```python
from build123d import *

# Parameters (mm, degrees)
CYLINDER_R        = 3.15
CYLINDER_DEPTH    = 10
CYLINDER001_R     = 6.5
CYLINDER001_DEPTH = 3
BOX_W             = 24
BOX_H             = 8
BOX_DEPTH         = 20
CHAMFER_SIZE      = 5
BOX001_W          = 7.8
BOX001_H          = 1
BOX001_DEPTH      = 20
FILLET_R          = 1
CHAMFER001_SIZE   = 0.4


with BuildPart() as cylinder:
    # Cylinder → Cylinder (new body)
    with BuildSketch(Plane(origin=(0, 0, 10), x_dir=(1, 0, 0), z_dir=(0, 1, 0))):
        Circle(CYLINDER_R)
    extrude(amount=CYLINDER_DEPTH)


with BuildPart() as fusion:
    # Cylinder001 → Cylinder001 (new body)
    with BuildSketch(Plane(origin=(0, 0, 10), x_dir=(1, 0, 0), z_dir=(0, 1, 0))):
        Circle(CYLINDER001_R)
    extrude(amount=CYLINDER001_DEPTH)

    # Fusion: union Cylinder
    add(cylinder.part)


with BuildPart() as chamfer_body:
    # Box → Box (new body)
    with BuildSketch(Plane(origin=(-12, 0, 0), x_dir=(1, 0, 0), z_dir=(0, 0, 1))):
        with Locations((12, 4)):
            Rectangle(BOX_W, BOX_H)
    extrude(amount=BOX_DEPTH)

    # Chamfer
    chamfer_edges = [chamfer_body.edges().sort_by_distance(p)[0] for p in [
        (-12, 4, 20),
        (12, 4, 20),
    ]]
    chamfer(chamfer_edges, length=CHAMFER_SIZE)


with BuildPart() as chamfer001:
    # Box001 → Box001 (new body)
    with BuildSketch(Plane(origin=(-3.9, 8, 0), x_dir=(1, 0, 0), z_dir=(0, 0, 1))):
        with Locations((3.9, 0.5)):
            Rectangle(BOX001_W, BOX001_H)
    extrude(amount=BOX001_DEPTH)

    # Fusion001: union Chamfer body
    add(chamfer_body.part)

    # Cut: cut Fusion
    add(fusion.part, mode=Mode.SUBTRACT)

    # Fillet
    fillet_edges = [chamfer001.edges().sort_by_distance(p)[0] for p in [
        (-12, 4, 15),
        (-7, 4, 20),
        (12, 4, 15),
        (7, 4, 20),
    ]]
    fillet(fillet_edges, radius=FILLET_R)

    # Chamfer001
    chamfer001_edges = [chamfer001.edges().sort_by_distance(p)[0] for p in [
        (-12, 0, 7.292893),
        (-12, 4, 0),
        (12, 0, 7.292893),
        (0, 0, 0),
        (-11.92388, 0, 14.96847),
        (-9.5, 0, 17.5),
        (-6.96847, 0, 19.92388),
        (0, 0, 20),
        (6.96847, 0, 19.92388),
        (9.5, 0, 17.5),
        (11.92388, 0, 14.96847),
        (-7.95, 8, 0),
        (12, 4, 0),
        (7.95, 8, 0),
        (-3.9, 8.5, 0),
        (0, 9, 0),
        (3.9, 8.5, 0),
    ]]
    chamfer(chamfer001_edges, length=CHAMFER001_SIZE)


solid = chamfer001.part
```
Could you check a few things on this model? Use its own coordinates, in mm. A direction names the side the tool comes from. Coordinates: 2 decimals unless noted, no trailing zeros. Order: outer loops, then holes, each group sorted by start corner. A loop starts at its lowest first (then second) coordinate and runs counter-clockwise, first axis right, second up. Notation, with made-up numbers: M 58,32.5 L 111,32.5 A16 ccw 111,47.5 Z; hole C -13,6 d9. An arc over 180 degrees is marked long. Use a Markdown table: item, result. Add a question column.
Q1. I want a section at D-D on z = 2.75. List the corners of the cut face in (x, y) for me, then the cut area to 3 significant figures.
Q2. If I drill on L1, parallel to Z at x = 0, y = 2; L2, parallel to Z at x = 0, y = 7.2; L3, parallel to Y at x = 4.25, z = 7, over which ranges is the centre line in solid material (lowest first)?
Q3. We'd pull the mould along X, two halves only. Please class faces 4 (the flat face through (3.9, 8.5, 10.1)), 5 (the cylindrical face through (-0.41, 5.958, 6.877)), 6 (the flat face through (-3.9, 8.5, 10.1)): pulls with the +X half, pulls with the -X half, needs draft (parallel to the pull), parting line crosses it, or undercut.
Q4. Which directions (+Z, -Z, +X, -X, +Y, -Y) give clear straight access to the entire face, cutting with the end or side of a thin tool? Please do faces 1 (the cylindrical face through (-1.409, 1.479, 16.345)), 2 (the flat face through (-8, 8, 10)), 3 (the flat face through (8, 8, 10)).
Q5. I want a section at B-B on y = 4.75. List the corners of the cut face in (x, z) for me, then the cut area to 3 significant figures.
Q6. I want a section at C-C on x = 0. List the corners of the cut face in (y, z) for me.
Q7. I want a section at A-A on z = 10. List the corners of the cut face in (x, y) for me, then the cut area to 3 significant figures.
Q8. I'm going to push flat-ended pins straight in: pin 1 (0.5 mm diameter, centred on y = 8.5, z = 7.5, fed in from +X); pin 2 (5 mm diameter, centred on x = 0, z = 10, fed in from -Y); pin 3 (6 mm diameter, centred on x = -7, z = 16, fed in from +Y); pin 4 (1.5 mm diameter, centred on x = -0.5, z = 6, fed in from -Y). Where does each tip first touch, or does it pass through?
Checked values:
| question | item | result |
|---|---|---|
| 1 | outline | M -12,0.4 L -11.6,0 L 11.6,0 L 12,0.4 L 12,8 L 3.9,8 L 3.9,9 L -3.9,9 L -3.9,8 L -12,8 Z |
| 1 | area | 200 mm² |
| 2 | L1 | 0 to 3.5, 16.5 to 20 |
| 2 | L2 | 0 to 6.85, 13.15 to 20 |
| 2 | L3 | 3 to 8 |
| 3 | face 4 | pulls with the +X half |
| 3 | face 5 | undercut |
| 3 | face 6 | pulls with the -X half |
| 4 | face 1 | -Y |
| 4 | face 2 | +Z, -Z, -X, +Y |
| 4 | face 3 | +Z, -Z, +X, +Y |
| 5 | outline | M -12,0.4 L -11.6,0 L 11.6,0 L 12,0.4 L 12,14.59 A1 ccw 11.71,15.29 L 7.29,19.71 A1 ccw 6.59,20 L -6.59,20 A1 ccw -7.29,19.71 L -11.71,15.29 A1 ccw -12,14.59 Z; hole C 0,10 d6.3 |
| 5 | area | 424 mm² |
| 6 | outline | M 0,0.4 L 0.4,0 L 8.6,0 L 9,0.4 L 9,6.85 L 3,6.85 L 3,3.5 L 0,3.5 Z; M 0,16.5 L 3,16.5 L 3,13.15 L 9,13.15 L 9,20 L 0.4,20 L 0,19.6 Z |
| 7 | outline | M -12,0.4 L -11.6,0 L -6.5,0 L -6.5,3 L -3.15,3 L -3.15,9 L -3.9,9 L -3.9,8 L -12,8 Z; M 3.15,3 L 6.5,3 L 6.5,0 L 11.6,0 L 12,0.4 L 12,8 L 3.9,8 L 3.9,9 L 3.15,9 Z |
| 7 | area | 123 mm² |
| 8 | pin 1 | x = 3.9 |
| 8 | pin 2 | through |
| 8 | pin 3 | y = 8 |
| 8 | pin 4 | y = 3 |
